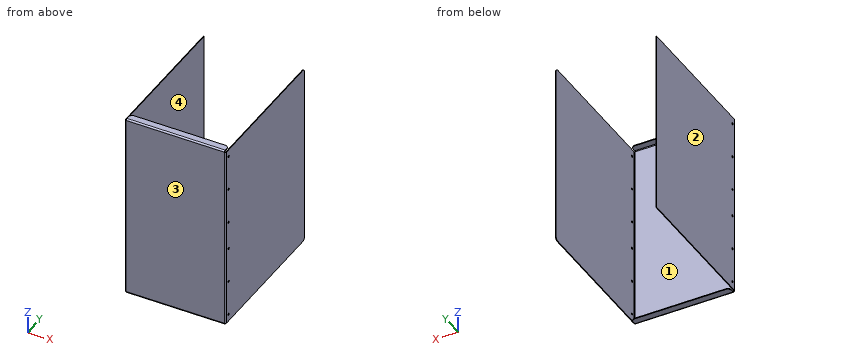
```python
from build123d import *

# Parameters (mm, degrees)
SKETCH1_W                    = 142
SKETCH1_H                    = 260
BASE_FLANGE1_DEPTH           = 1
EDGE_FLANGE1_STRIP_W         = 6
EDGE_FLANGE1_STRIP_H         = 1
EDGE_FLANGE1_STRIP_CUT_DEPTH = 260
EDGE_FLANGE1_DEPTH           = 260
EDGE_FLANGE2_STRIP_W         = 6
EDGE_FLANGE2_STRIP_H         = 1
EDGE_FLANGE2_STRIP_CUT_DEPTH = 260
EDGE_FLANGE2_DEPTH           = 260
EDGE_FLANGE2_FLAT_DEPTH      = 1
EDGE_FLANGE4_DEPTH           = 138
EDGE_FLANGE4_START           = 1
EDGE_FLANGE4_FLAT_DEPTH      = 1
SKETCH12_R                   = 1.5
CUT_EXTRUDE1_DEPTH           = 157
EDGE_FLANGE5_DEPTH           = 138
EDGE_FLANGE5_START           = 1
EDGE_FLANGE5_FLAT_DEPTH      = 1


# Sheet-metal steps are written as plain solids
with BuildPart() as part:
    # Sketch1 → Base-Flange1 (new body)
    with BuildSketch(Plane(origin=(0, 0, 0), x_dir=(1, 0, 0), z_dir=(0, 1, 0))):
        with Locations((71, 130)):
            Rectangle(SKETCH1_W, SKETCH1_H)
    extrude(amount=-BASE_FLANGE1_DEPTH)

    # Edge-Flange1 strip (across the edge) → Edge-Flange1 strip cut (cut)
    with BuildSketch(Plane.XY.offset(-260)):
        with Locations((-1, -0.5)):
            Rectangle(EDGE_FLANGE1_STRIP_W, EDGE_FLANGE1_STRIP_H)
    extrude(amount=EDGE_FLANGE1_STRIP_CUT_DEPTH, mode=Mode.SUBTRACT)

    # Edge-Flange1 section (across the edge) → Edge-Flange1 (add)
    with BuildSketch(Plane.XY.offset(-260)):
        with BuildLine():
            Line((0, 1), (0, 200))
            Line((0, 200), (1, 200))
            Line((1, 200), (1, 1))
            ThreePointArc((1, 1), (1.292893219, 0.292893219), (2, 0))
            Line((2, 0), (2, -1))
            ThreePointArc((2, -1), (0.585786438, -0.414213562), (0, 1))
        make_face()
    extrude(amount=EDGE_FLANGE1_DEPTH)

    # Edge-Flange2 strip (across the edge) → Edge-Flange2 strip cut (cut)
    with BuildSketch(Plane(origin=(142, 0, 0), x_dir=(-1, 0, 0), z_dir=(0, 0, -1))):
        with Locations((-1, -0.5)):
            Rectangle(EDGE_FLANGE2_STRIP_W, EDGE_FLANGE2_STRIP_H)
    extrude(amount=EDGE_FLANGE2_STRIP_CUT_DEPTH, mode=Mode.SUBTRACT)

    # Edge-Flange2 bend section (across the edge) → Edge-Flange2 (add)
    with BuildSketch(Plane(origin=(142, 0, 0), x_dir=(-1, 0, 0), z_dir=(0, 0, -1))):
        with BuildLine():
            Line((0, 1), (1, 1))
            ThreePointArc((1, 1), (1.292893219, 0.292893219), (2, 0))
            Line((2, 0), (2, -1))
            ThreePointArc((2, -1), (0.585786438, -0.414213562), (0, 1))
        make_face()
    extrude(amount=EDGE_FLANGE2_DEPTH)

    # Edge-Flange2 profile (on flange) → Edge-Flange2 flat (add)
    with BuildSketch(Plane(origin=(142, 0, 0), x_dir=(0, 0, -1), z_dir=(1, 0, 0))):
        with BuildLine():
            ThreePointArc((5, 200), (1.464466094, 198.535533906), (0, 195))
            Line((0, 195), (0, 1))
            Line((0, 1), (260, 1))
            Line((260, 1), (260, 195))
            ThreePointArc((260, 195), (258.535533906, 198.535533906), (255, 200))
            Line((255, 200), (5, 200))
        make_face()
    extrude(amount=-EDGE_FLANGE2_FLAT_DEPTH)

    # Edge-Flange4 bend section (across the edge) → Edge-Flange4 (add)
    with BuildSketch(Plane(origin=(140, 0, -261), x_dir=(0, 0, 1), z_dir=(-1, 0, 0))):
        with BuildLine():
            Line((-1, 1), (0, 1))
            ThreePointArc((0, 1), (0.292893219, 0.292893219), (1, 0))
            Line((1, 0), (1, -1))
            ThreePointArc((1, -1), (-0.414213562, -0.414213562), (-1, 1))
        make_face()
    extrude(amount=EDGE_FLANGE4_DEPTH)

    # Edge-Flange4 profile (on flange) → Edge-Flange4 flat (add)
    with BuildSketch(Plane(origin=(0, 0, -261), x_dir=(-1, 0, 0), z_dir=(0, 0, -1)).offset(EDGE_FLANGE4_START)):
        with BuildLine():
            Line((-7, 10), (-135, 10))
            ThreePointArc((-135, 10), (-138.535533906, 8.535533906), (-140, 5))
            Line((-140, 5), (-140, 1))
            Line((-140, 1), (-2, 1))
            Line((-2, 1), (-2, 5))
            ThreePointArc((-2, 5), (-3.464466094, 8.535533906), (-7, 10))
        make_face()
    extrude(amount=-EDGE_FLANGE4_FLAT_DEPTH)

    # Sketch12 → Cut-Extrude1 (cut)
    with BuildSketch(Plane.ZY):
        with Locations(Location((-110, 6, 0), (0, 0, 270))):
            Circle(SKETCH12_R)
        with Locations(Location((-60, 6, 0), (0, 0, 270))):
            Circle(SKETCH12_R)
        with Locations(Location((-10, 6, 0), (0, 0, 270))):
            Circle(SKETCH12_R)
        with Locations(Location((-150, 6, 0), (0, 0, 270))):
            Circle(SKETCH12_R)
        with Locations(Location((-200, 6, 0), (0, 0, 270))):
            Circle(SKETCH12_R)
        with Locations(Location((-250, 6, 0), (0, 0, 270))):
            Circle(SKETCH12_R)
    extrude(amount=-CUT_EXTRUDE1_DEPTH, mode=Mode.SUBTRACT)

    # Edge-Flange5 bend section (across the edge) → Edge-Flange5 (add)
    with BuildSketch(Plane(origin=(2, 0, 1), x_dir=(0, 0, -1), z_dir=(1, 0, 0))):
        with BuildLine():
            Line((-1, 1), (0, 1))
            ThreePointArc((0, 1), (0.292893219, 0.292893219), (1, 0))
            Line((1, 0), (1, -1))
            ThreePointArc((1, -1), (-0.414213562, -0.414213562), (-1, 1))
        make_face()
    extrude(amount=EDGE_FLANGE5_DEPTH)

    # Edge-Flange5 profile (on flange) → Edge-Flange5 flat (add)
    with BuildSketch(Plane.XY.offset(1).offset(EDGE_FLANGE5_START)):
        with BuildLine():
            Line((135, 10), (7, 10))
            ThreePointArc((7, 10), (3.464466094, 8.535533906), (2, 5))
            Line((2, 5), (2, 1))
            Line((2, 1), (140, 1))
            Line((140, 1), (140, 5))
            ThreePointArc((140, 5), (138.535533906, 8.535533906), (135, 10))
        make_face()
    extrude(amount=-EDGE_FLANGE5_FLAT_DEPTH)


solid = part.part
```
Verification items for the finished model (mm, model axes). Face numbers are marked on the shaded views. A direction names the side the tool comes from. Coordinates: 2 decimals unless noted, no trailing zeros. Loops run counter-clockwise (first coordinate to the right, second up) from the corner with the lowest first, then second, coordinate; pieces in that order, holes last. Notation, with made-up numbers: (0, 44.25) - (17, 44.25) arc R19 cw to (17, 48.25) - close; hole circle Ø9 at (58, -29). An arc over 180 degrees is marked (long way). Answer as a JSON object with one key per item and string values.
(1) Mould release check, pull along Z, two halves, no side actions. Record for the marked faces 1 and 2: pulls with the +Z half, pulls with the -Z half, needs draft (parallel to the pull), parting line crosses it, or undercut.
Response:
{"face 1": "undercut", "face 2": "needs draft"}
(2) Cross-section at A-A, the plane y = 134. Record the boundary of the cut face in (x, z).
Response:
{"outline": "(0, -260) - (1, -260) - (1, 0) - (0, 0) - close; (141, -260) - (142, -260) - (142, 0) - (141, 0) - close"}
(3) Access from +Z, -Z, +X, -X, +Y, -Y to the whole of each face (thin tool, end or side, straight path). Record for the marked faces 3 and 4.
Response:
{"face 3": "+Z, -Z, +X, -X, -Y", "face 4": "+Z, -Z, +Y"}
(4) Go/stop test with flat-tipped pins: pin 1 Ø1.8 at (y, z) = (6, -250) entering from +X; pin 2 Ø1.6 at (x, y) = (141, 88.5) entering from +Z; pin 3 Ø0.5 at (x, z) = (101.5, 1.5) entering from +Y; pin 4 Ø1.5 at (x, z) = (122, -139.5) entering from +Y. Record where each tip stops, or that it passes through.
Response:
{"pin 1": "passes through", "pin 2": "stops at z = 0", "pin 3": "stops at y = 10", "pin 4": "stops at y = 0"}
(5) Cross-section at C-C, the plane z = -193.5. Record the boundary of the cut face in (x, y).
Response:
{"outline": "(0, 1) arc R2 ccw to (2, -1) - (140, -1) arc R2 ccw to (142, 1) - (142, 200) - (141, 200) - (141, 1) arc R1 cw to (140, 0) - (2, 0) arc R1 cw to (1, 1) - (1, 200) - (0, 200) - close"}
(6) Cross-section at B-B, the plane x = 67. Record the boundary of the cut face in (y, z), then the cut area to 3 significant figures.
Response:
{"outline": "(-1, -260) arc R2 ccw to (1, -262) - (10, -262) - (10, -261) - (1, -261) arc R1 cw to (0, -260) - (0, 0) arc R1 cw to (1, 1) - (10, 1) - (10, 2) - (1, 2) arc R2 ccw to (-1, 0) - close", "area": "283 mm²"}
(7) Scan lines: line 1 along X through (y, z) = (95, -80.5); line 2 along Y through (x, z) = (141.7, -250); line 3 along Y through (x, z) = (125.5, -38.5). Record each from-to range of solid material in increasing order.
Response:
{"line 1": "x = 0 to 1, 141 to 142", "line 2": "y = -0.05 to 4.5, 7.5 to 200", "line 3": "y = -1 to 0"}
